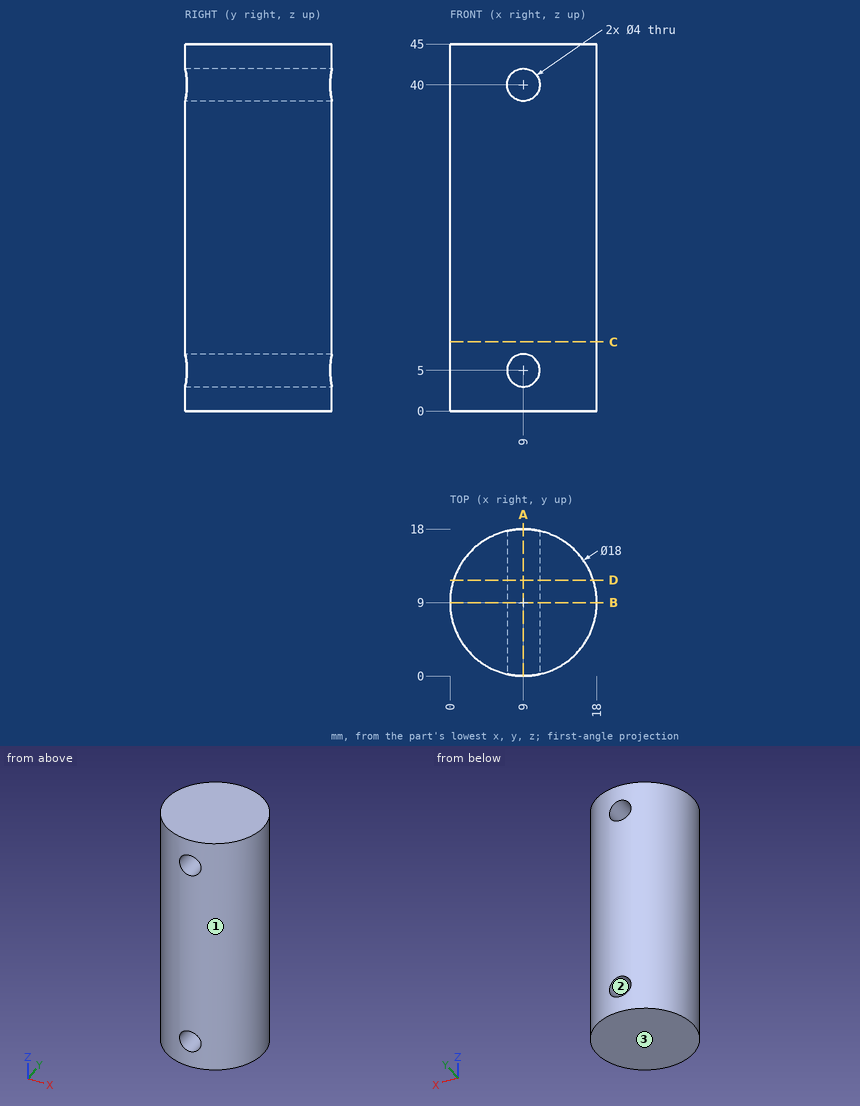
Check sheet for the drawn part. Datum: minimum x, y, z corner. Units: mm. Give positions to 0.01 mm unless a question says otherwise; leave off trailing zeros. Loops run counter-clockwise (first coordinate to the right, second up) from the corner with the lowest first, then second, coordinate; pieces in that order, holes last. Notation, with made-up numbers: M 8.5,-21 L 23.5,-21 A19 ccw 23.5,-7 Z; hole C 89,-23.75 d9. An arc over 180 degrees is marked long. Return JSON: item names as keys, results as strings.
1) Section check B-B, the plane y = 9. Enter the section's corners in (x, z).
Findings:
{"outline": "M 0,0 L 18,0 L 18,45 L 0,45 Z; hole C 9,5 d4; hole C 9,40 d4"}
2) Section check C-C, the plane z = 8.5. Enter the section's corners in (x, y), and give its area (3 significant figures).
Findings:
{"outline": "C 9,9 d18", "area": "254 mm2"}
3) Mould release check, pull along X, two halves, no side actions. Record for the marked faces 1, 2 and 3: released by +X, released by -X, zero draft, split by the parting line, or undercut.
Findings:
{"face 1": "split by the parting line", "face 2": "undercut", "face 3": "zero draft"}
4) Section check A-A, the plane x = 9. Enter the section's corners in (y, z).
Findings:
{"outline": "M 0,0 L 18,0 L 18,3 L 0,3 Z; M 0,7 L 18,7 L 18,38 L 0,38 Z; M 0,42 L 18,42 L 18,45 L 0,45 Z"}
5) Material ranges on L1, parallel to Z at x = 9.75, y = 5; L2, parallel to X at y = 4.25, z = 40; L3, parallel to X at y = 12.25, z = 41, recorded low to high. Write a range as [from, to].
Findings:
{"L1": "z = [0, 3.15], [6.85, 38.15], [41.85, 45]", "L2": "x = [1.36, 7], [11, 16.64]", "L3": "x = [0.61, 7.27], [10.73, 17.39]"}
6) Gauge pin test, flat ends, axial feed: P1, Ø10, axis at y = 16, z = 35, coming from the +X side; P2, Ø10, axis at y = 15, z = 18, coming from the -X side; P3, Ø6, axis at x = 2.5, z = 13.5, coming from the -Y side; P4, Ø2.5, axis at x = 9, z = 40, coming from the -Y side. Record the tip position at first contact, or that the pin passes through.
Findings:
{"P1": "stops at x = 17.77", "P2": "stops at x = 0.06", "P3": "stops at y = 0.71", "P4": "passes through"}
7) Section check D-D, the plane y = 11.75. Enter the section's corners in (x, z).
Findings:
{"outline": "M 0.43,0 L 17.57,0 L 17.57,45 L 0.43,45 Z; hole C 9,5 d4; hole C 9,40 d4"}
